```python
from build123d import *

# Parameters (mm, degrees)
F0_R     = 47.625
F0_R_2   = 3.5687
F1_DEPTH = 6.35


with BuildPart() as f1:
    # F0 (on Right) → F1 (new body)
    with BuildSketch(Plane.YZ):
        Circle(F0_R)
        with Locations((-29.1846, -29.1846)):
            Circle(F0_R_2, mode=Mode.SUBTRACT)
        with Locations((29.1846, -29.1846)):
            Circle(F0_R_2, mode=Mode.SUBTRACT)
        with Locations((-29.1846, 29.1846)):
            Circle(F0_R_2, mode=Mode.SUBTRACT)
        with Locations((29.1846, 29.1846)):
            Circle(F0_R_2, mode=Mode.SUBTRACT)
    extrude(amount=-F1_DEPTH)


solid = f1.part
```
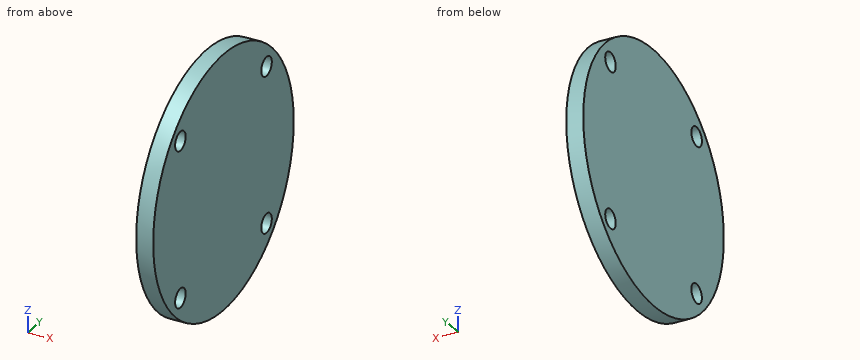
Verification items for the finished model (mm, model axes). Coordinates: 2 decimals unless noted, no trailing zeros. Loops run counter-clockwise (first coordinate to the right, second up) from the corner with the lowest first, then second, coordinate; pieces in that order, holes last. Notation, with made-up numbers: (27, -21.75) -> (32, -21.75) arc R18 ccw to (32, -6.75) -> close; hole circle Ø1 at (-27, 27). An arc over 180 degrees is marked (long way). Put each result on its own line as item: value.
1. Section check C-C, the plane y = 20.5. Record the boundary of the cut face in (x, z).
Result set:
outline: (-6.35, -42.99) -> (0, -42.99) -> (0, 42.99) -> (-6.35, 42.99) -> close
2. Section check B-B, the plane x = -4.5. Record the boundary of the cut face in (y, z) (3 decimals).
Result set:
outline: circle Ø95.25 at (0, 0); hole circle Ø7.137 at (-29.185, -29.185); hole circle Ø7.137 at (-29.185, 29.185); hole circle Ø7.137 at (29.185, -29.185); hole circle Ø7.137 at (29.185, 29.185)
3. Thickness scan on line 1 (Z direction, x = -5.25, y = 0.5); line 2 (Y direction, x = -4.5, z = 28); line 3 (Y direction, x = -6, z = -2). Record the ranges inside material, lowest first.
Result set:
line 1: z = -47.62 to 47.62
line 2: y = -38.52 to -32.55, -25.82 to 25.82, 32.55 to 38.52
line 3: y = -47.58 to 47.58
4. Section check A-A, the plane z = -27. Record the boundary of the cut face in (x, y), then the cut area to 3 significant figures.
Result set:
outline: (-6.35, -39.23) -> (0, -39.23) -> (0, -32.01) -> (-6.35, -32.01) -> close; (-6.35, -26.36) -> (0, -26.36) -> (0, 26.36) -> (-6.35, 26.36) -> close; (-6.35, 32.01) -> (0, 32.01) -> (0, 39.23) -> (-6.35, 39.23) -> close
area: 427 mm^2
